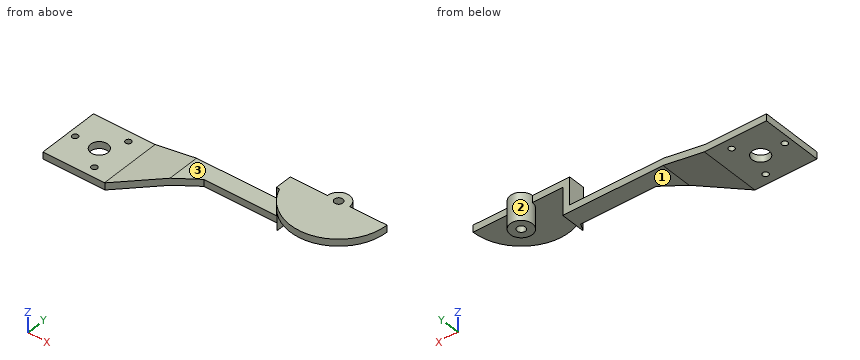
from build123d import *

# Parameters (mm, degrees)
ESQUISSE1_R             = 6
ESQUISSE1_R_2           = 4.25
BASE_EXTRUSION_DEPTH    = 60
ENL_V_MAT_EXTRU_1_DEPTH = 396.094925303
ENL_V_MAT_EXTRU_2_DEPTH = 10
ENL_V_MAT_EXTRU_3_DEPTH = 40
ESQUISSE5_R             = 12.5
ENL_V_MAT_EXTRU_4_DEPTH = 389.099214119
ESQUISSE6_R             = 16
ESQUISSE6_R_2           = 6
ENL_V_MAT_EXTRU_5_DEPTH = 10


with BuildPart() as part:
    # Esquisse1 → Base-Extrusion (new body)
    with BuildSketch(Plane.XY):
        with BuildLine():
            Line((380, 45), (326, 45))
            ThreePointArc((326, 45), (310, 61), (294, 45))
            Line((294, 45), (-45, 45))
            Line((-45, 45), (-45, -45))
            Line((-45, -45), (45, -45))
            Line((45, -45), (135, 20))
            Line((135, 20), (244.616515847, 20))
            ThreePointArc((244.616515847, 20), (322.711335675, -23.836196477), (380, 45))
        make_face()
        with Locations(Location((310, 45, 0), (0, 0, 180))):
            Circle(ESQUISSE1_R, mode=Mode.SUBTRACT)
        with Locations(Location((-35, 0, 0), (0, 0, 180))):
            Circle(ESQUISSE1_R_2, mode=Mode.SUBTRACT)
        with Locations(Location((17.5, 30.310889132, 0), (0, 0, 180))):
            Circle(ESQUISSE1_R_2, mode=Mode.SUBTRACT)
        with Locations(Location((17.5, -30.310889132, 0), (0, 0, 180))):
            Circle(ESQUISSE1_R_2, mode=Mode.SUBTRACT)
    extrude(amount=BASE_EXTRUSION_DEPTH)

    # Esquisse2 → Enlèv. mat.-Extru.1 (cut, through all)
    with BuildSketch(Plane(origin=(0, 45, 0), x_dir=(-1, 0, 0), z_dir=(0, 1, 0))):
        Polygon((-294, 50), (-294, 10), (-326, 10), (-326, 50), (-380, 50), (-380, 0), (-45, 0), (-105, 10), (-250, 10), (-250, 50), align=None)
        Polygon((-240, 60), (-240, 20), (-104.172374697, 20), (-44.172374697, 10), (45, 10), (45, 60), align=None)
    extrude(amount=-ENL_V_MAT_EXTRU_1_DEPTH, mode=Mode.SUBTRACT)

    # Esquisse3 → Enlèv. mat.-Extru.2 (cut)
    with BuildSketch(Plane(origin=(0, 0, 0), x_dir=(-1, 0, 0), z_dir=(0, 0, -1))):
        with BuildLine():
            Line((-304, 45), (-294, 45))
            ThreePointArc((-294, 45), (-310, 61), (-326, 45))
            Line((-326, 45), (-316, 45))
            ThreePointArc((-316, 45), (-310, 51), (-304, 45))
        make_face()
    extrude(amount=-ENL_V_MAT_EXTRU_2_DEPTH, mode=Mode.SUBTRACT)

    # Esquisse4 → Enlèv. mat.-Extru.3 (cut)
    with BuildSketch(Plane(origin=(0, 0, 10), x_dir=(-1, 0, 0), z_dir=(0, 0, -1))):
        with BuildLine():
            ThreePointArc((-326, -23.14690015), (-310, -25), (-294, -23.14690015))
            Line((-294, -23.14690015), (-294, 45))
            ThreePointArc((-294, 45), (-310, 29), (-326, 45))
            Line((-326, 45), (-326, -23.14690015))
        make_face()
    extrude(amount=-ENL_V_MAT_EXTRU_3_DEPTH, mode=Mode.SUBTRACT)

    # Esquisse5 → Enlèv. mat.-Extru.4 (cut, through all)
    with BuildSketch(Plane.XY.offset(10)):
        Circle(ESQUISSE5_R)
    extrude(amount=-ENL_V_MAT_EXTRU_4_DEPTH, mode=Mode.SUBTRACT)

    # Esquisse6 → Enlèv. mat.-Extru.5 (cut)
    with BuildSketch(Plane(origin=(0, 0, 10), x_dir=(-1, 0, 0), z_dir=(0, 0, -1))):
        with Locations((-310, 45)):
            Circle(ESQUISSE6_R)
        with Locations((-310, 45)):
            Circle(ESQUISSE6_R_2, mode=Mode.SUBTRACT)
    extrude(amount=-ENL_V_MAT_EXTRU_5_DEPTH, mode=Mode.SUBTRACT)


solid = part.part
Check sheet for the modelled part. Datum: model origin and axes. Units: mm. Face numbers are marked on the shaded views. A direction names the side the tool comes from. Round coordinates to 2 decimals unless told otherwise and drop trailing zeros. Loops run counter-clockwise (first coordinate to the right, second up) from the corner with the lowest first, then second, coordinate; pieces in that order, holes last. Notation, with made-up numbers: (76.5, 36.5) -> (91.5, 36.5) arc R27 ccw to (91.5, 74.5) -> close; hole circle Ø3 at (69, 45). An arc over 180 degrees is marked (long way). Put each result on its own line as item: value. Start each with the question number.
1. Scan lines: probe 1 along Y at (x, z) = (310, 33); probe 2 along Y at (x, z) = (-35, 4.75); probe 3 along Y at (x, z) = (243.5, 49). Record each from-to range of solid material in increasing order.
2. Section check D-D (z = 5). Enter the section's corners in (x, y), plus the area to 3 significant figures.
3. Section check B-B (z = 30). Enter the section's corners in (x, y).
4. Access from +Z, -Z, +X, -X, +Y, -Y to the whole of each face (thin tool, end or side, straight path). Record for the marked faces 1, 2 and 3.
5. Gauge pin test, flat ends, axial feed: pin 1 (5 mm diameter, centred on x = -35, y = 0, fed in from -Z); pin 2 (6 mm diameter, centred on x = 296.5, z = 29.5, fed in from +Y); pin 3 (6 mm diameter, centred on x = 40.5, y = 18, fed in from +Z); pin 4 (14 mm diameter, centred on x = 310, y = 45, fed in from -Z). Record the tip position at first contact, or that the pin passes through.
6. Section check A-A (x = 0). Enter the section's corners in (y, z), plus the area to 3 significant figures.
7. Section check C-C (x = 310). Enter the section's corners in (y, z), plus the area to 3 significant figures.
Findings:
1. probe 1: y = 29 to 39, 51 to 61
1. probe 2: y = -45 to -4.25, 4.25 to 45
1. probe 3: y = 20 to 45
2. outline: (-45, -45) -> (45, -45) -> (75, -23.33) -> (75, 45) -> (-45, 45) -> close; hole circle Ø8.5 at (-35, 0); hole circle Ø25 at (0, 0); hole circle Ø8.5 at (17.5, -30.31); hole circle Ø8.5 at (17.5, 30.31)
2. area: 9,810 mm^2
3. outline: (240, 20) -> (244.62, 20) arc R70 ccw to (250, 8.94) -> (250, 45) -> (240, 45) -> close; circle Ø32 at (310, 45); hole circle Ø12 at (310, 45)
4. face 1: -Z, +X, +Y, -Y
4. face 2: -Z
4. face 3: +Z, -X, +Y, -Y
5. pin 1: passes through
5. pin 2: stops at y = 57.07
5. pin 3: stops at z = 10
5. pin 4: stops at z = 20
6. outline: (-45, 0) -> (-12.5, 0) -> (-12.5, 10) -> (-45, 10) -> close; (12.5, 0) -> (45, 0) -> (45, 10) -> (12.5, 10) -> close
6. area: 650 mm^2
7. outline: (-25, 50) -> (29, 50) -> (29, 20) -> (39, 20) -> (39, 60) -> (-25, 60) -> close; (51, 20) -> (61, 20) -> (61, 60) -> (51, 60) -> close
7. area: 1,340 mm^2
